Autodesk Inventor part; units mm, degrees
ref_plane "YZ Plane" through (0, 0, 0) normal (1, 0, 0) x (0, 1, 0)
ref_plane "XZ Plane" through (0, 0, 0) normal (0, 1, 0) x (-1, 0, 0)
ref_plane "XY Plane" through (0, 0, 0) normal (0, 0, 1) x (1, 0, 0)
sketch "Sketch1" plane through (0, 0, 0) normal (0, 1, 0) x (-1, 0, 0)
  line L0 (0, 3.1754) -> (2.75, 1.5877)
  line L1 (2.75, 1.5877) -> (2.75, -1.5877)
  line L2 (2.75, -1.5877) -> (0, -3.1754)
  line L3 (0, -3.1754) -> (-2.75, -1.5877)
  line L4 (-2.75, -1.5877) -> (-2.75, 1.5877)
  line L5 (-2.75, 1.5877) -> (0, 3.1754)
  circle A0 centre (0, 0) radius 1.5
  point P0 (2.75, 0)
  dimension "d0" = 5.5
  dimension "d1" = 3
extrude "Extrusion1" add sketch "Sketch1" along normal blind 2.2
properties part number "Tuerca_M3" material "Stainless Steel"
The listing builds one solid part. Answer for the finished solid, in the listing's coordinates (mm). Give positions to 0.01 mm unless a question says otherwise; leave off trailing zeros. Loops run counter-clockwise (first coordinate to the right, second up) from the corner with the lowest first, then second, coordinate; pieces in that order, holes last. Notation, with made-up numbers: (84.25, 69.25) - (127.25, 69.25) arc R32 cw to (127.25, 102.25) - close; hole circle Ø8 at (54, -38). An arc over 180 degrees is marked (long way). Return JSON: item names as keys, results as strings. Group by question number.
1. Given pin 1 Ø1.8 at (x, z) = (0, 0) entering from -Y, flat-ended and moving along its own axis, determine where the tip first touches the part or whether it passes through.
2. Find section C-C (z = 0). Write down the section's boundary in (x, y).
3. Find section B-B (z = 1.25). Write down the section's boundary in (x, y), then the cut area to 3 significant figures.
4. Find section D-D (x = -2). Write down the section's boundary in (y, z).
5. Determine the mould class of faces 1 (the cylindrical face through (1.5, 1.08, -0.07)), 2 (the flat face through (-2.75, 1, 0)), 3 (the flat face through (1.394, 1.085, 2.37)) for opening direction X: pulls with the +X half, pulls with the -X half, needs draft (parallel to the pull), parting line crosses it, or undercut.
6. Straight lines are drawn through the part: line 1 (Z direction, x = 1.15, y = 2.15); line 2 (X direction, y = 0.55, z = 1); line 3 (X direction, y = 1.75, z = -0.75). For each, find the intervals that lie inside material, in ascending order. Write a range as [from, to].
7. Find section A-A (y = 1.75). Write down the section's boundary in (x, z), then the cut area to 3 significant figures.
Verdict:
{
 "1": {"pin 1": "passes through"},
 "2": {"outline": "(-2.75, 0) - (-1.5, 0) - (-1.5, 2.2) - (-2.75, 2.2) - close; (1.5, 0) - (2.75, 0) - (2.75, 2.2) - (1.5, 2.2) - close"},
 "3": {"outline": "(-2.75, 0) - (-0.83, 0) - (-0.83, 2.2) - (-2.75, 2.2) - close; (0.83, 0) - (2.75, 0) - (2.75, 2.2) - (0.83, 2.2) - close", "area": "8.45 mm^2"},
 "4": {"outline": "(0, -2.02) - (2.2, -2.02) - (2.2, 2.02) - (0, 2.02) - close"},
 "5": {"face 1": "undercut", "face 2": "pulls with the -X half", "face 3": "pulls with the +X half"},
 "6": {"line 1": "z = [-2.51, -0.96], [0.96, 2.51]", "line 2": "x = [-2.75, -1.12], [1.12, 2.75]", "line 3": "x = [-2.75, -1.3], [1.3, 2.75]"},
 "7": {"outline": "(-2.75, -1.59) - (0, -3.18) - (2.75, -1.59) - (2.75, 1.59) - (0, 3.18) - (-2.75, 1.59) - close; hole circle Ø3 at (0, 0)", "area": "19.1 mm^2"}
}
